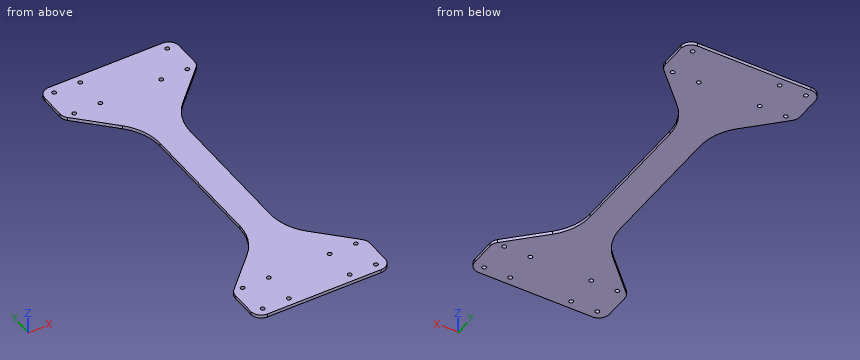
```python
from build123d import *

# Parameters (mm, degrees)
BOSS_EXTRUDE1_DEPTH = 3.175
CUT_EXTRUDE1_DEPTH  = 10
SKETCH3_R           = 2.0193
BOSS_EXTRUDE2_DEPTH = 3.175
FILLET1_R           = 10
FILLET2_R           = 50


with BuildPart() as part:
    # Sketch1 → Boss-Extrude1 (new body)
    with BuildSketch(Plane.XY):
        Polygon((165.934536959, -16.66935), (157.315236959, -8.05005), (115.359952094, -8.05005), (89.959952094, -8.05005), (48.004667228, -8.05005), (39.385367228, -16.66935), (39.385367228, -40.05005), (39.385367228, -52.41105), (165.934536959, -56.67505), (165.934536959, -42.05005), align=None)
        with BuildLine():
            ThreePointArc((47.685367228, -44.38075), (49.704667228, -46.40005), (47.685367228, -48.41935))
            ThreePointArc((47.685367228, -48.41935), (45.666067228, -46.40005), (47.685367228, -44.38075))
        make_face(mode=Mode.SUBTRACT)
        with BuildLine():
            ThreePointArc((47.685367228, -12.63075), (49.704667228, -14.65005), (47.685367228, -16.66935))
            ThreePointArc((47.685367228, -16.66935), (45.666067228, -14.65005), (47.685367228, -12.63075))
        make_face(mode=Mode.SUBTRACT)
        with BuildLine():
            ThreePointArc((73.085367228, -44.38075), (75.104667228, -46.40005), (73.085367228, -48.41935))
            ThreePointArc((73.085367228, -48.41935), (71.066067228, -46.40005), (73.085367228, -44.38075))
        make_face(mode=Mode.SUBTRACT)
        with BuildLine():
            ThreePointArc((73.085367228, -12.63075), (75.104667228, -14.65005), (73.085367228, -16.66935))
            ThreePointArc((73.085367228, -16.66935), (71.066067228, -14.65005), (73.085367228, -12.63075))
        make_face(mode=Mode.SUBTRACT)
        with BuildLine():
            ThreePointArc((132.234536959, -44.38075), (134.253836959, -46.40005), (132.234536959, -48.41935))
            ThreePointArc((132.234536959, -48.41935), (130.215236959, -46.40005), (132.234536959, -44.38075))
        make_face(mode=Mode.SUBTRACT)
        with BuildLine():
            ThreePointArc((132.234536959, -12.63075), (134.253836959, -14.65005), (132.234536959, -16.66935))
            ThreePointArc((132.234536959, -16.66935), (130.215236959, -14.65005), (132.234536959, -12.63075))
        make_face(mode=Mode.SUBTRACT)
        with BuildLine():
            ThreePointArc((157.634536959, -44.38075), (159.653836959, -46.40005), (157.634536959, -48.41935))
            ThreePointArc((157.634536959, -48.41935), (155.615236959, -46.40005), (157.634536959, -44.38075))
        make_face(mode=Mode.SUBTRACT)
        with BuildLine():
            ThreePointArc((157.634536959, -12.63075), (159.653836959, -14.65005), (157.634536959, -16.66935))
            ThreePointArc((157.634536959, -16.66935), (155.615236959, -14.65005), (157.634536959, -12.63075))
        make_face(mode=Mode.SUBTRACT)
        Polygon((115.359952094, -8.05005), (157.315236959, -8.05005), (115.359952094, 33.905234866), align=None)
        Polygon((89.959952094, -8.05005), (115.359952094, -8.05005), (115.359952094, 33.905234866), (115.359952094, 203.394265134), (115.359952094, 245.34955), (89.959952094, 245.34955), (89.959952094, 203.394265134), (89.959952094, 33.905234866), align=None)
        Polygon((48.004667228, -8.05005), (89.959952094, -8.05005), (89.959952094, 33.905234866), align=None)
        Polygon((89.959952094, 245.34955), (115.359952094, 245.34955), (157.315236959, 245.34955), (165.934536959, 253.96885), (165.934536959, 279.34955), (165.934536959, 293.97455), (39.385367228, 289.71055), (39.385367228, 277.34955), (39.385367228, 253.96885), (48.004667228, 245.34955), align=None)
        with BuildLine():
            ThreePointArc((47.685367228, 253.96885), (49.704667228, 251.94955), (47.685367228, 249.93025))
            ThreePointArc((47.685367228, 249.93025), (45.666067228, 251.94955), (47.685367228, 253.96885))
        make_face(mode=Mode.SUBTRACT)
        with BuildLine():
            ThreePointArc((47.685367228, 285.71885), (49.704667228, 283.69955), (47.685367228, 281.68025))
            ThreePointArc((47.685367228, 281.68025), (45.666067228, 283.69955), (47.685367228, 285.71885))
        make_face(mode=Mode.SUBTRACT)
        with BuildLine():
            ThreePointArc((73.085367228, 253.96885), (75.104667228, 251.94955), (73.085367228, 249.93025))
            ThreePointArc((73.085367228, 249.93025), (71.066067228, 251.94955), (73.085367228, 253.96885))
        make_face(mode=Mode.SUBTRACT)
        with BuildLine():
            ThreePointArc((73.085367228, 285.71885), (75.104667228, 283.69955), (73.085367228, 281.68025))
            ThreePointArc((73.085367228, 281.68025), (71.066067228, 283.69955), (73.085367228, 285.71885))
        make_face(mode=Mode.SUBTRACT)
        with BuildLine():
            ThreePointArc((132.234536959, 253.96885), (134.253836959, 251.94955), (132.234536959, 249.93025))
            ThreePointArc((132.234536959, 249.93025), (130.215236959, 251.94955), (132.234536959, 253.96885))
        make_face(mode=Mode.SUBTRACT)
        with BuildLine():
            ThreePointArc((157.634536959, 253.96885), (159.653836959, 251.94955), (157.634536959, 249.93025))
            ThreePointArc((157.634536959, 249.93025), (155.615236959, 251.94955), (157.634536959, 253.96885))
        make_face(mode=Mode.SUBTRACT)
        with BuildLine():
            ThreePointArc((157.634536959, 285.71885), (159.653836959, 283.69955), (157.634536959, 281.68025))
            ThreePointArc((157.634536959, 281.68025), (155.615236959, 283.69955), (157.634536959, 285.71885))
        make_face(mode=Mode.SUBTRACT)
        Polygon((115.359952094, 245.34955), (115.359952094, 203.394265134), (157.315236959, 245.34955), align=None)
        Polygon((48.004667228, 245.34955), (89.959952094, 203.394265134), (89.959952094, 245.34955), align=None)
    extrude(amount=BOSS_EXTRUDE1_DEPTH)

    # Sketch2 → Cut-Extrude1 (cut)
    with BuildSketch(Plane.XY.offset(3.175)):
        Polygon((84.385367228, -52.41105), (39.385367228, -52.41105), (165.934536959, -56.67505), (165.934536959, -52.41105), (120.934536959, -52.41105), align=None)
        Polygon((120.934536959, 289.71055), (165.934536959, 289.71055), (165.934536959, 293.97455), (39.385367228, 289.71055), (84.385367228, 289.71055), align=None)
    extrude(amount=-CUT_EXTRUDE1_DEPTH, mode=Mode.SUBTRACT)

    # Sketch3 → Boss-Extrude2 (add)
    with BuildSketch(Plane.XY.offset(3.175)):
        Polygon((37.385367228, -15.840922875), (37.385367228, -54.41105), (167.934536959, -54.41105), (167.934536959, -15.840922875), (117.359952094, 34.73366199), (117.359952094, 202.56583801), (167.934536959, 253.140422875), (167.934536959, 291.71055), (37.385367228, 291.71055), (37.385367228, 253.140422875), (87.959952094, 202.56583801), (87.959952094, 34.73366199), align=None)
        with Locations((132.234536959, -46.40005)):
            Circle(SKETCH3_R, mode=Mode.SUBTRACT)
        with Locations((132.234536959, -14.65005)):
            Circle(SKETCH3_R, mode=Mode.SUBTRACT)
        with Locations((47.685367228, -14.65005)):
            Circle(SKETCH3_R, mode=Mode.SUBTRACT)
        with Locations((47.685367228, -46.40005)):
            Circle(SKETCH3_R, mode=Mode.SUBTRACT)
        with Locations((73.085367228, -46.40005)):
            Circle(SKETCH3_R, mode=Mode.SUBTRACT)
        with Locations((73.085367228, -14.65005)):
            Circle(SKETCH3_R, mode=Mode.SUBTRACT)
        with Locations((157.634536959, -14.65005)):
            Circle(SKETCH3_R, mode=Mode.SUBTRACT)
        with Locations((157.634536959, -46.40005)):
            Circle(SKETCH3_R, mode=Mode.SUBTRACT)
        with Locations((132.234536959, 251.94955)):
            Circle(SKETCH3_R, mode=Mode.SUBTRACT)
        with Locations((73.085367228, 251.94955)):
            Circle(SKETCH3_R, mode=Mode.SUBTRACT)
        with Locations((157.634536959, 251.94955)):
            Circle(SKETCH3_R, mode=Mode.SUBTRACT)
        with Locations((47.685367228, 251.94955)):
            Circle(SKETCH3_R, mode=Mode.SUBTRACT)
        with Locations((47.685367228, 283.69955)):
            Circle(SKETCH3_R, mode=Mode.SUBTRACT)
        with Locations((73.085367228, 283.69955)):
            Circle(SKETCH3_R, mode=Mode.SUBTRACT)
        with Locations((157.634536959, 283.69955)):
            Circle(SKETCH3_R, mode=Mode.SUBTRACT)
    extrude(amount=-BOSS_EXTRUDE2_DEPTH)

    # Fillet1
    fillet1_edges = [part.edges().sort_by_distance(p)[0] for p in [
        (37.385367228, -54.41105, 1.5875),
        (167.934536959, -54.41105, 1.5875),
        (167.934536959, -15.840922875, 1.5875),
        (167.934536959, 253.140422875, 1.5875),
        (167.934536959, 291.71055, 1.5875),
        (37.385367228, 291.71055, 1.5875),
        (37.385367228, 253.140422875, 1.5875),
        (37.385367228, -15.840922875, 1.5875),
    ]]
    fillet(fillet1_edges, radius=FILLET1_R)

    # Fillet2
    fillet2_edges = [part.edges().sort_by_distance(p)[0] for p in [
        (117.359952094, 34.73366199, 1.5875),
        (117.359952094, 202.56583801, 1.5875),
        (87.959952094, 202.56583801, 1.5875),
        (87.959952094, 34.73366199, 1.5875),
    ]]
    fillet(fillet2_edges, radius=FILLET2_R)


solid = part.part
```
Part model, mm, in its own coordinate system. Coordinates: 2 decimals unless noted, no trailing zeros. Loops run counter-clockwise (first coordinate to the right, second up) from the corner with the lowest first, then second, coordinate; pieces in that order, holes last. Notation, with made-up numbers: (37.25, 77) - (55.25, 77) arc R28 ccw to (55.25, 99) - close; hole circle Ø4 at (74, -35.5). An arc over 180 degrees is marked (long way). Write item = value, one per line. Start each with the question number.
Item 1: Cut at A-A, the plane x = 125. Give the cut face in (y, z) (3 decimals), and give its area (3 significant figures).
Item 2: Cut at B-B, the plane x = 85. Give the cut face in (y, z) (3 decimals), and give its area (3 significant figures).
Item 3: Wall check: L1, parallel to X at y = -15, z = 2.1; L2, parallel to Y at x = 121, z = 0.6; L3, parallel to X at y = -14, z = 2.85. Give the ranges that are in metal, low to high. Write a range as from..to.
Item 4: Cut at C-C, the plane y = 82.5. Give the cut face in (x, z) (3 decimals).
Item 5: Cut at D-D, the plane z = 2.5. State how many separate pieces and enclosed holes the cut face has, and give its area (3 significant figures).
The answers:
q1.outline = (-54.411, 0) - (28.881, 0) - (28.881, 3.175) - (-54.411, 3.175) - close; (208.419, 0) - (291.711, 0) - (291.711, 3.175) - (208.419, 3.175) - close
q1.area = 529 mm2
q2.outline = (-54.411, 0) - (38.496, 0) - (38.496, 3.175) - (-54.411, 3.175) - close; (198.803, 0) - (291.711, 0) - (291.711, 3.175) - (198.803, 3.175) - close
q2.area = 590 mm2
q3.L1 = 38.72..45.7, 49.67..71.1, 75.07..130.25, 134.22..155.65, 159.62..166.6
q3.L2 = -54.41..36.72, 200.58..291.71
q3.L3 = 39.37..45.77, 49.6..71.17, 75..130.32, 134.15..155.72, 159.55..165.95
q4.outline = (87.96, 0) - (117.36, 0) - (117.36, 3.175) - (87.96, 3.175) - close
q5.separate_pieces = 1
q5.enclosed_holes = 15
q5.area = 23,000 mm2
